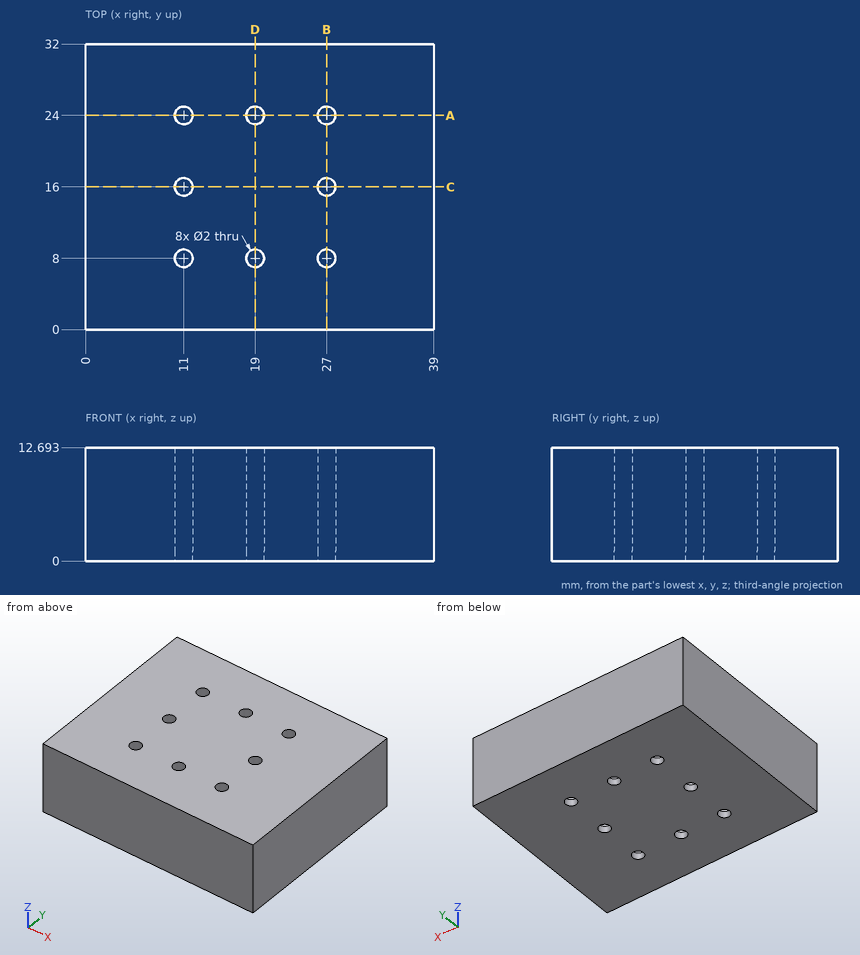
Source: three-view drawing plus pictorial views. Frame: mm from the lowest corner of the part. Give positions to 0.01 mm unless a question says otherwise; leave off trailing zeros. Loops run counter-clockwise (first coordinate to the right, second up) from the corner with the lowest first, then second, coordinate; pieces in that order, holes last. Notation, with made-up numbers: (19.25, 4.25) -> (23.25, 4.25) arc R12 ccw to (23.25, 15.25) -> close; hole circle Ø11 at (-3.5, 58.25). An arc over 180 degrees is marked (long way). Use a Markdown table: item, result. Add a question column.
(1) Section query D-D (x = 19). Output: boundary loops of the cut face in (y, z).
(2) First-contact query: pin 1 Ø4 at (x, y) = (10.5, 17.5) entering from -Z. Flat tip, straight axial feed; report the tip coordinate or a pass-through.
(3) Section query A-A (y = 24). Output: boundary loops of the cut face in (x, z), then the cut area to 3 significant figures.
(4) Ray query, line 1 (X direction, y = 16, z = 0.7); line 2 (X direction, y = 24, z = 0.7); line 3 (Y direction, x = 11, z = 0.65). Return the intervals inside material, ascending.
(5) Section query B-B (x = 27). Output: boundary loops of the cut face in (y, z).
(6) Section query C-C (y = 16). Output: boundary loops of the cut face in (x, z).
Checked values:
| question | item | result |
|---|---|---|
| 1 | outline | (0, 0) -> (7, 0) -> (7, 12.69) -> (0, 12.69) -> close; (9, 0) -> (23, 0) -> (23, 12.69) -> (9, 12.69) -> close; (25, 0) -> (32, 0) -> (32, 12.69) -> (25, 12.69) -> close |
| 2 | pin 1 | z = 0 |
| 3 | outline | (0, 0) -> (10, 0) -> (10, 12.69) -> (0, 12.69) -> close; (12, 0) -> (18, 0) -> (18, 12.69) -> (12, 12.69) -> close; (20, 0) -> (26, 0) -> (26, 12.69) -> (20, 12.69) -> close; (28, 0) -> (39, 0) -> (39, 12.69) -> (28, 12.69) -> close |
| 3 | area | 419 mm^2 |
| 4 | line 1 | 0 to 10, 12 to 26, 28 to 39 |
| 4 | line 2 | 0 to 10, 12 to 18, 20 to 26, 28 to 39 |
| 4 | line 3 | 0 to 7, 9 to 15, 17 to 23, 25 to 32 |
| 5 | outline | (0, 0) -> (7, 0) -> (7, 12.69) -> (0, 12.69) -> close; (9, 0) -> (15, 0) -> (15, 12.69) -> (9, 12.69) -> close; (17, 0) -> (23, 0) -> (23, 12.69) -> (17, 12.69) -> close; (25, 0) -> (32, 0) -> (32, 12.69) -> (25, 12.69) -> close |
| 6 | outline | (0, 0) -> (10, 0) -> (10, 12.69) -> (0, 12.69) -> close; (12, 0) -> (26, 0) -> (26, 12.69) -> (12, 12.69) -> close; (28, 0) -> (39, 0) -> (39, 12.69) -> (28, 12.69) -> close |
